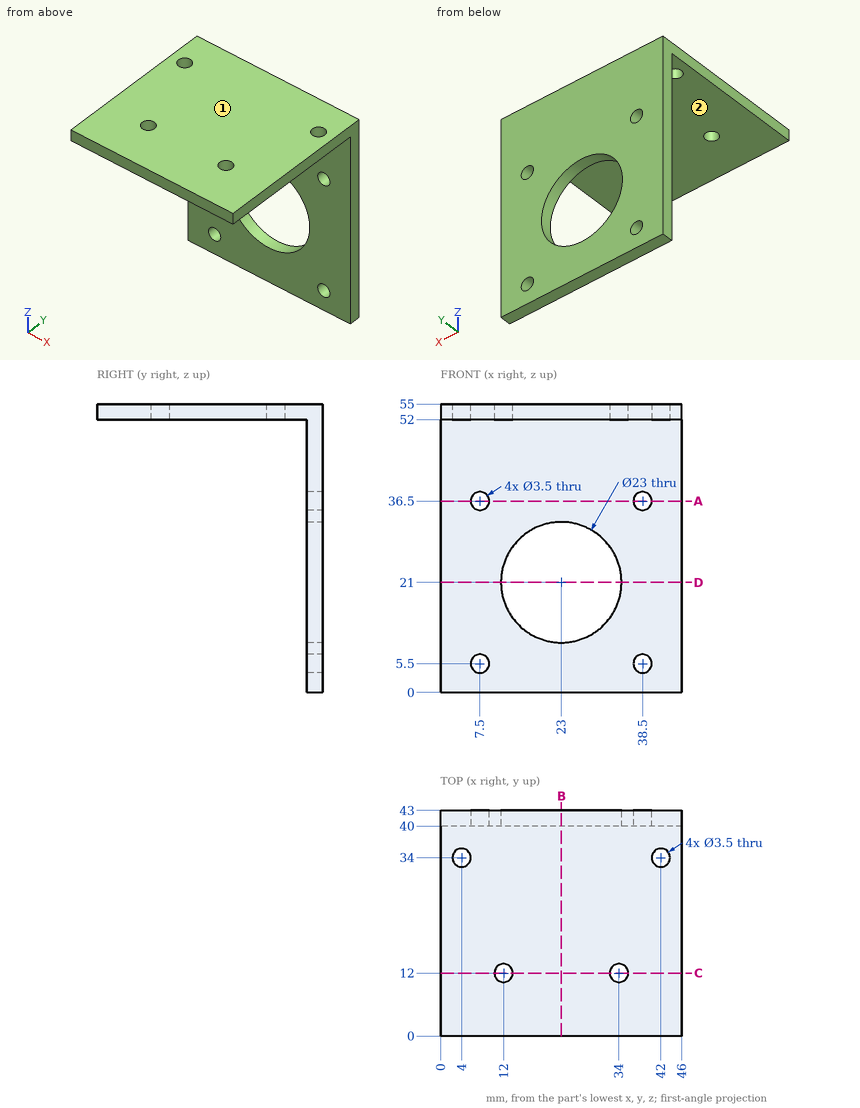
Check sheet for the drawn part. Datum: minimum x, y, z corner. Units: mm. A direction names the side the tool comes from. Coordinates: 2 decimals unless noted, no trailing zeros. Loops run counter-clockwise (first coordinate to the right, second up) from the corner with the lowest first, then second, coordinate; pieces in that order, holes last. Notation, with made-up numbers: M 38.5,56.25 L 84.5,56.25 A26 ccw 84.5,95.25 Z; hole C 54,64.5 d6. An arc over 180 degrees is marked long. Answer as a JSON object with one key per item and string values.
1. Sectioned sample at B-B on x = 23. Record the cut outline in (y, z), and give its area (3 significant figures).
Outcome:
{"outline": "M 0,52 L 40,52 L 40,32.5 L 43,32.5 L 43,55 L 0,55 Z; M 40,0 L 43,0 L 43,9.5 L 40,9.5 Z", "area": "216 mm²"}
2. Sectioned sample at A-A on z = 36.5. Record the cut outline in (x, y).
Outcome:
{"outline": "M 0,40 L 5.75,40 L 5.75,43 L 0,43 Z; M 9.25,40 L 36.75,40 L 36.75,43 L 9.25,43 Z; M 40.25,40 L 46,40 L 46,43 L 40.25,43 Z"}
3. Depth check by flat-ended pin: P1, Ø23, axis at x = 27, z = 24, coming from the -Y side; P2, Ø12, axis at x = 40.5, y = 26, coming from the -Z side. Enter the tip coordinate at first touch or a pass-through.
Outcome:
{"P1": "y = 40", "P2": "z = 52"}
4. Scan lines: L1, parallel to Z at x = 7.5, y = 42.05; L2, parallel to Y at x = 42, z = 52.8; L3, parallel to Y at x = 41, z = 16. Record each from-to range of solid material in increasing order. Write a range as from..to.
Outcome:
{"L1": "0..3.75, 7.25..34.75, 38.25..55", "L2": "0..32.25, 35.75..43", "L3": "40..43"}
5. Sectioned sample at D-D on z = 21. Record the cut outline in (x, y).
Outcome:
{"outline": "M 0,40 L 11.5,40 L 11.5,43 L 0,43 Z; M 34.5,40 L 46,40 L 46,43 L 34.5,43 Z"}
6. Sectioned sample at C-C on y = 12. Record the cut outline in (x, z).
Outcome:
{"outline": "M 0,52 L 10.25,52 L 10.25,55 L 0,55 Z; M 13.75,52 L 32.25,52 L 32.25,55 L 13.75,55 Z; M 35.75,52 L 46,52 L 46,55 L 35.75,55 Z"}
7. Access from +Z, -Z, +X, -X, +Y, -Y to the whole of each face (thin tool, end or side, straight path). Record for the marked faces 1 and 2.
Outcome:
{"face 1": "+Z, +X, -X, +Y, -Y", "face 2": "-Z, +X, -X, -Y"}
